Check sheet for the modelled part. Datum: model origin and axes. Units: mm. A direction names the side the tool comes from. Round coordinates to 2 decimals unless told otherwise and drop trailing zeros. Write each loop counter-clockwise with the first axis right and the second up, starting at its lowest first coordinate (ties: lowest second). Pieces come first, ordered by that corner, then holes. Notation, with made-up numbers: M 16.25,12 L 23.25,12 A19 ccw 23.25,45 Z; hole C 82,78 d9. An arc over 180 degrees is marked long. Put each result on its own line as item: value.
```python
from build123d import *

# Parameters (mm, degrees)
SALIENTE_EXTRUIR1_DEPTH = 18
CROQUIS3_W              = 23
CROQUIS3_H              = 16
CORTAR_EXTRUIR1_DEPTH   = 1
REDONDEO1_R             = 1


with BuildPart() as part:
    # Croquis2 → Saliente-Extruir1 (new body)
    with BuildSketch(Plane(origin=(0, 0, 0), x_dir=(1, 0, 0), z_dir=(0, 1, 0))):
        Polygon((0, 130), (0, 0), (23, 0), (23, 50), (14, 50), (14, 130), align=None)
    extrude(amount=SALIENTE_EXTRUIR1_DEPTH)

    # Croquis3 → Cortar-Extruir1 (cut)
    with BuildSketch(Plane.XY):
        with Locations((11.5, 8)):
            Rectangle(CROQUIS3_W, CROQUIS3_H)
    extrude(amount=-CORTAR_EXTRUIR1_DEPTH, mode=Mode.SUBTRACT)

    # Redondeo1
    redondeo1_edges = [part.edges().sort_by_distance(p)[0] for p in [
        (0, 18, -65),
        (11.5, 18, 0),
        (23, 18, -25),
    ]]
    fillet(redondeo1_edges, radius=REDONDEO1_R)


solid = part.part
```
1. Depth check by flat-ended pin: pin 1 Ø3 at (x, y) = (18, 2.5) entering from +Z; pin 2 Ø4 at (y, z) = (12.5, -108.5) entering from +X; pin 3 Ø0.8 at (x, z) = (12.5, -0.5) entering from -Y. Enter the tip coordinate at first touch or a pass-through.
Computed values:
pin 1: stops at z = -1
pin 2: stops at x = 14
pin 3: stops at y = 16
2. Cross-section at A-A (x = 18.5). Enter the section's corners in (y, z), then the cut area to 3 significant figures.
Computed values:
outline: M 0,-50 L 18,-50 L 18,-1 A1 ccw 17,0 L 16,0 L 16,-1 L 0,-1 Z
area: 884 mm2
3. Cross-section at B-B (y = 12.75). Enter the section's corners in (x, z).
Computed values:
outline: M 0,-130 L 14,-130 L 14,-50 L 23,-50 L 23,-1 L 0,-1 Z
4. Access from +Z, -Z, +X, -X, +Y, -Y to the whole of each face (thin tool, end or side, straight path). Record for faces 1 (the flat face through (19, 9, -50)), 2 (the flat face through (11, 8, -1)), 3 (the flat face through (0, 8, -66)).
Computed values:
face 1: -Z, +X, +Y, -Y
face 2: +Z, +X, -X, -Y
face 3: +Z, -Z, -X, +Y, -Y
5. Cross-section at C-C (z = -93.5). Enter the section's corners in (x, y).
Computed values:
outline: M 0,0 L 14,0 L 14,18 L 1,18 A1 ccw 0,17 Z
6. Scan lines: probe 1 along Z at (x, y) = (18.75, 12.25); probe 2 along X at (y, z) = (12.75, -96.5); probe 3 along Z at (x, y) = (6, 3). Record each from-to range of solid material in increasing order.
Computed values:
probe 1: z = -50 to -1
probe 2: x = 0 to 14
probe 3: z = -130 to -1
